```python
from build123d import *

# Parameters (mm, degrees)
F3_DEPTH = 1.27


with BuildPart() as f1:
    # F0 (on Front) → F1 (revolve)
    with BuildSketch(Plane.XZ):
        Polygon((1.905, 2.352728), (0, 2.352728), (0, -7.807272), (1.1303, -7.807272), (1.1303, 0.447728), (1.905, 0.447728), align=None)
    revolve(axis=Axis((0, 0, -2.727272), (0, 0, -1)))

    # F2 (on face) → F3 (cut)
    with BuildSketch(Plane.XY.offset(2.352728)):
        Polygon((-1.176285, 0.679128), (-1.176285, -0.679128), (0, -1.358256), (1.176285, -0.679128), (1.176285, 0.679128), (0, 1.358256), align=None)
    extrude(amount=-F3_DEPTH, mode=Mode.SUBTRACT)


solid = f1.part
```
Geometry: final body of the model. Coordinates: model frame, mm. A direction names the side the tool comes from. Coordinates: 2 decimals unless noted, no trailing zeros. Write each loop counter-clockwise with the first axis right and the second up, starting at its lowest first coordinate (ties: lowest second). Pieces come first, ordered by that corner, then holes. Notation, with made-up numbers: M 7,46.25 L 25,46.25 A14 cw 25,68.25 Z; hole C 49.5,63.5 d5. An arc over 180 degrees is marked long. Answer as CSV lines item,"result". Start each with the question number.
Q1. Line query: line 1 (X direction, y = -0.1, z = 1.25); line 2 (Z direction, x = 0.6, y = -0.1); line 3 (Y direction, x = -0.55, z = 1.25). Output: solid intervals per line, ascending. Write a range as from..to.
Q2. Mould query, pull axis Y, two halves, no side actions, for faces 1 (the flat face through (1.176, 0, 2)), 2 (the flat face through (0, 0, -7.807)), 3 (the cylindrical face through (-0.41, 1.86, 1.41)). Classes: released by +Y, released by -Y, zero draft, split by the parting line, or undercut.
Q3. Cut plane B-B on z = -2. Return the cut outline in (x, y).
Q4. Pin query (flat end, axial travel): P1, Ø0.7, axis at x = 0, y = 0.5, coming from the +Z side. Return the tip coordinate at first contact, or that it passes through.
Q5. Cut plane C-C on x = 0.6. Return the cut outline in (y, z).
Q6. Cut plane A-A on y = 0. Return the cut outline in (x, z) (3 decimals), then the cut area to 3 significant figures.
Q7. Reachability of faces 4 (the flat face through (-1, -1, 2.353)), 5 (the flat face through (0.6, 1.01, 1.73)), 6 (the flat face through (-1, 1, 0.448)) from +Z, -Z, +X, -X, +Y, -Y: full face, straight path, thin tool, end or side. Return the list, or none.
Q8. Cut plane D-D on x = -1.5. Return the cut outline in (y, z).
Findings below:
1,line 1,"x = -1.9..-1.18, 1.18..1.9"
1,line 2,"z = -7.81..1.08"
1,line 3,"y = -1.82..-1.04, 1.04..1.82"
2,face 1,"undercut"
2,face 2,"zero draft"
2,face 3,"split by the parting line"
3,outline,"C 0,0 d2.26"
4,P1,"stops at z = 1.08"
5,outline,"M -1.81,0.45 L -0.96,0.45 L -0.96,-7.81 L 0.96,-7.81 L 0.96,0.45 L 1.81,0.45 L 1.81,2.35 L 1.01,2.35 L 1.01,1.08 L -1.01,1.08 L -1.01,2.35 L -1.81,2.35 Z"
6,outline,"M -1.905,0.448 L -1.13,0.448 L -1.13,-7.807 L 1.13,-7.807 L 1.13,0.448 L 1.905,0.448 L 1.905,2.353 L 1.176,2.353 L 1.176,1.083 L -1.176,1.083 L -1.176,2.353 L -1.905,2.353 Z"
6,area,"22.9 mm2"
7,face 4,"+Z, +X, -X, +Y, -Y"
7,face 5,"+Z"
7,face 6,"-Z"
8,outline,"M -1.17,0.45 L 1.17,0.45 L 1.17,2.35 L -1.17,2.35 Z"
